Here's how the part is built. I have some questions about the finished solid (model axes, mm). A direction names the side the tool comes from. Coordinates: 2 decimals unless noted, no trailing zeros. Write each loop counter-clockwise with the first axis right and the second up, starting at its lowest first coordinate (ties: lowest second). Pieces come first, ordered by that corner, then holes. Notation, with made-up numbers: (-4.5, 27) -> (37.5, 27) arc R14 ccw to (37.5, 49) -> close; hole circle Ø8 at (-5, 76.5). An arc over 180 degrees is marked (long way). Answer in a Markdown table with one row per item. Add a question column.
from build123d import *

# Parameters (mm, degrees)
SKETCH1_W           = 40
SKETCH1_H           = 40
BOSS_EXTRUDE1_DEPTH = 40
CUT_EXTRUDE1_DEPTH  = 40
CUT_EXTRUDE3_DEPTH  = 20


with BuildPart() as part:
    # Sketch1 → Boss-Extrude1 (new body)
    with BuildSketch(Plane.XY):
        with Locations((20, 20)):
            Rectangle(SKETCH1_W, SKETCH1_H)
    extrude(amount=BOSS_EXTRUDE1_DEPTH)

    # Sketch2 → Cut-Extrude1 (cut)
    with BuildSketch(Plane.XY.offset(40)):
        Polygon((0, 0), (20, 40), (0, 40), align=None)
    extrude(amount=-CUT_EXTRUDE1_DEPTH, mode=Mode.SUBTRACT)

    # Sketch3 → Cut-Extrude3 (cut)
    with BuildSketch(Plane(origin=(40, 0, 0), x_dir=(0, 0, -1), z_dir=(1, 0, 0))):
        Polygon((-40, 40), (-40, 0), (-30, 20), align=None)
        Polygon((-30, 20), (-40, 0), (-20, 0), align=None)
        Polygon((-10, 20), (0, 0), (0, 40), align=None)
        Polygon((-10, 20), (-20, 0), (0, 0), align=None)
    extrude(amount=-CUT_EXTRUDE3_DEPTH, mode=Mode.SUBTRACT)


solid = part.part
Q1. Imagine slicing it at C-C on x = 8. Please give me the cut outline in (y, z).
Q2. Imagine slicing it at A-A on y = 14. Please give me the cut outline in (x, z).
Q3. Imagine slicing it at D-D on z = 14.5. Please give me the cut outline in (x, y), plus the area to 3 significant figures.
Q4. I'm going to push flat-ended pins straight in: P1, Ø1.5, axis at x = 16, z = 21, coming from the -Y side; P2, Ø4, axis at x = 8, z = 32.5, coming from the +Y side; P3, Ø3, axis at x = 34, y = 20.5, coming from the +Z side; P4, Ø6, axis at x = 26, z = 31, coming from the -Y side. Where does each tip first touch, or does it pass through?
Q5. I need wall thicknesses on line 1 (Z direction, x = 31.5, y = 2); line 2 (X direction, y = 27, z = 25.5); line 3 (X direction, y = 16, z = 6). Which ranges of each line are inside material? Lowest first, please. Write a range as [from, to].
Q6. For faces 1 (the flat face through (20, 11, 35)), 2 (the flat face through (30, 40, 20)), 3 (the flat face through (30, 20, 10)), which set-ups out of +Z, -Z, +X, -X, +Y, -Y let a thin tool reach every point of the face, with its end or its side?
Q7. Imagine slicing it at B-B on z = 3.5. Please give me the cut outline in (x, y), plus the area to 3 significant figures.
Result sheet:
| question | item | result |
|---|---|---|
| 1 | outline | (0, 0) -> (16, 0) -> (16, 40) -> (0, 40) -> close |
| 2 | outline | (7, 0) -> (20, 0) -> (20, 13) -> (40, 13) -> (40, 27) -> (20, 27) -> (20, 40) -> (7, 40) -> close |
| 3 | outline | (0, 0) -> (20, 0) -> (20, 11) -> (40, 11) -> (40, 40) -> (20, 40) -> close |
| 3 | area | 980 mm^2 |
| 4 | P1 | stops at y = 0 |
| 4 | P2 | stops at y = 20 |
| 4 | P3 | stops at z = 31 |
| 4 | P4 | stops at y = 16 |
| 5 | line 1 | z = [19, 21] |
| 5 | line 2 | x = [13.5, 40] |
| 5 | line 3 | x = [8, 20] |
| 6 | face 1 | +Z, +X, -Y |
| 6 | face 2 | +Z, -Z, +X, -X, +Y |
| 6 | face 3 | -Z, +X, -Y |
| 7 | outline | (0, 0) -> (20, 0) -> (20, 33) -> (40, 33) -> (40, 40) -> (20, 40) -> close |
| 7 | area | 540 mm^2 |
